from build123d import *

# Parameters (mm, degrees)
SKETCH_1_R = 6


with BuildPart() as part:
    # По траектории1: sweep along a path in Эскиз2
    with BuildLine(Plane.XY) as sweep_1_path:
        Line((-6, 0), (-6, 34.113207547))
        ThreePointArc((-6, 34.113207547), (-10.100505063, 44.012702484), (-20, 48.113207547))
        Line((-20, 48.113207547), (-27, 48.113207547))
        ThreePointArc((-27, 48.113207547), (-36.899494937, 52.213712611), (-41, 62.113207547))
        Line((-41, 62.113207547), (-41, 88.113207547))
    # Эскиз1 → По траектории1 (sweep)
    with BuildSketch(Plane(origin=(0, 0, 0), x_dir=(1, 0, 0), z_dir=(0, 1, 0))):
        with Locations((-6, 0)):
            Circle(SKETCH_1_R)
    sweep(path=sweep_1_path.line)


solid = part.part
Model file for the job. Use its own axes, mm. A direction names the side the tool comes from. Give positions to 0.01 mm unless a question says otherwise; leave off trailing zeros. Order: outer loops, then holes, each group sorted by start corner. A loop starts at its lowest first (then second) coordinate and runs counter-clockwise, first axis right, second up. Notation, with made-up numbers: (-17.5, 17) - (40.5, 17) arc R10 ccw to (40.5, 34) - close; hole circle Ø10 at (83, 22). An arc over 180 degrees is marked (long way). One line per item, written item: value.
Item 1: Pin check, flat tips, straight feed: pin 1 Ø5 at (y, z) = (70.5, 0) entering from +X; pin 2 Ø2 at (y, z) = (56, -1) entering from +X; pin 3 Ø6 at (x, z) = (-14, -2.5) entering from +Y. Stop position of each tip, or through.
Response values:
pin 1: x = -35
pin 2: x = -30.81
pin 3: y = 53.75
Item 2: Slice it at A-A (z = 0). List the corners of the cut face in (x, y), then the cut area to 3 significant figures.
Response values:
outline: (-47, 62.11) arc R20 ccw to (-27, 42.11) - (-20, 42.11) arc R8 cw to (-12, 34.11) - (-12, 0) - (0, 0) - (0, 34.11) arc R20 ccw to (-20, 54.11) - (-27, 54.11) arc R8 cw to (-35, 62.11) - (-35, 88.11) - (-47, 88.11) - close
area: 1,330 mm2
Item 3: Tool access for faces 1 (the cylindrical face through (-10.76, 17.3, 3.65)), 2 (the cylindrical face through (-47, 75, 0)), 3 (the cylindrical face through (-23.55, 42.12, -0.26)), 4 (the flat face through (-6, 0, 0)), 5 (the flat face through (-41, 88.113, 0)): list every direction of +Z, -Z, +X, -X, +Y, -Y with a clear straight run to the whole face (end or side of a thin tool).
Response values:
face 1: -Y
face 2: +Y
face 3: none
face 4: +Z, -Z, +X, -X, -Y
face 5: +Z, -Z, +X, -X, +Y
Item 4: Wall check: line 1 (Y direction, x = -15.5, z = 1.75); line 2 (X direction, y = 83.5, z = -1.75); line 3 (Y direction, x = -37, z = 4). Give the ranges that are in metal, low to high.
Response values:
line 1: 41.04 to 53.33
line 2: -46.74 to -35.26
line 3: 46.58 to 88.11
Item 5: Slice it at C-C (z = 5). List the corners of the cut face in (x, y), then the cut area to 3 significant figures.
Response values:
outline: (-44.32, 62.11) arc R17.32 ccw to (-27, 44.8) - (-20, 44.8) arc R10.68 cw to (-9.32, 34.11) - (-9.32, 0) - (-2.68, 0) - (-2.68, 34.11) arc R17.32 ccw to (-20, 51.43) - (-27, 51.43) arc R10.68 cw to (-37.68, 62.11) - (-37.68, 88.11) - (-44.32, 88.11) - close
area: 737 mm2
Item 6: Slice it at B-B (y = 23). List the corners of the cut face in (x, z).
Response values:
outline: circle Ø12 at (-6, 0)
